from build123d import *

# Parameters (mm, degrees)
SKETCH1_R               = 25
BOSS_EXTRUDE1_DEPTH     = 249.6
SKETCH2_R               = 24.61
BOSS_EXTRUDE2_DEPTH     = 200
CUT_EXTRUDE1_DEPTH      = 451.987982102
CUT_EXTRUDE1_DEPTH_BACK = 451.987982102
SKETCH3_R               = 11


with BuildPart() as part:
    # Sketch1 → Boss-Extrude1 (new body)
    with BuildSketch(Plane(origin=(0, 0, 0), x_dir=(1, 0, 0), z_dir=(0, 1, 0))):
        with Locations(Location((0, 0, 0), (0, 0, 270))):
            Circle(SKETCH1_R)
    extrude(amount=BOSS_EXTRUDE1_DEPTH)

    # Sketch2 → Boss-Extrude2 (add)
    with BuildSketch(Plane(origin=(0, 249.6, 0), x_dir=(1, 0, 0), z_dir=(0, 1, 0))):
        with Locations(Location((0, 0, 0), (0, 0, 270))):
            Circle(SKETCH2_R)
    extrude(amount=BOSS_EXTRUDE2_DEPTH)

    # Sketch3 → Cut-Extrude1 (cut, two sides: drawn at the far end of the back side and taken through both)
    with BuildSketch(Plane(origin=(0, 0, 0), x_dir=(0, 0, -1), z_dir=(1, 0, 0)).offset(-CUT_EXTRUDE1_DEPTH_BACK)):
        with Locations((0, 299.6)):
            Circle(SKETCH3_R)
        with Locations((0, 399.6)):
            Circle(SKETCH3_R)
    extrude(amount=CUT_EXTRUDE1_DEPTH + CUT_EXTRUDE1_DEPTH_BACK, mode=Mode.SUBTRACT)


solid = part.part
Work out the finished part from the listing and answer in its coordinate system (mm). Round coordinates to 2 decimals unless told otherwise and drop trailing zeros. Loops run counter-clockwise (first coordinate to the right, second up) from the corner with the lowest first, then second, coordinate; pieces in that order, holes last. Notation, with made-up numbers: (75, 13.5) - (98, 13.5) arc R15 cw to (98, 23.5) - close; hole circle Ø3 at (23.25, 29.25). An arc over 180 degrees is marked (long way). Use one line per item in the form item = value. Start each with the question number.
(1) Find section D-D on y = 299.6. Determine the outline of the cut face in (x, z), and give its area (3 significant figures).
(2) Find section C-C on z = -19. Determine the outline of the cut face in (x, y), and give its area (3 significant figures).
(3) Find section B-B on x = 0. Determine the outline of the cut face in (y, z).
(4) Find section A-A on z = 0. Determine the outline of the cut face in (x, y), and give its area (3 significant figures).
(5) Determine the mould class of faces 1 (the face through (-0.345, 295.387, -10.161)), 2 (the face through (-9.43, 348.2, 22.73)), 3 (the face through (-16.6, 249.6, 18.4)) for opening direction Z: +Z half, -Z half, draft (parallel to the pull), parting line (faces both ways), or undercut.
(6) Flat-ended cylindrical pins translate along their axes: P1, Ø1, axis at y = 164.5, z = -17, coming from the +X side; P2, Ø6, axis at y = 148.5, z = -12.5, coming from the -X side; P3, Ø2, axis at y = 186, z = -3, coming from the -X side. Find the tip coordinate at first contact, or state that the pin passes through.
(7) Consider line 1 (Y direction, x = -2.5, z = 0); line 2 (Z direction, x = -1, y = 299.6); line 3 (Y direction, x = 5.5, z = -2.5). Determine where each line is inside the solid, lowest interval first.
Answer list:
q1.outline = (-22.01, -11) arc R24.61 ccw to (22.01, -11) - close; (-22.01, 11) - (22.01, 11) arc R24.61 ccw to start
q1.area = 857 mm^2
q2.outline = (-16.25, 0) - (16.25, 0) - (16.25, 249.6) - (15.64, 249.6) - (15.64, 449.6) - (-15.64, 449.6) - (-15.64, 249.6) - (-16.25, 249.6) - close
q2.area = 14,400 mm^2
q3.outline = (0, -25) - (249.6, -25) - (249.6, -24.61) - (449.6, -24.61) - (449.6, 24.61) - (249.6, 24.61) - (249.6, 25) - (0, 25) - close; hole circle Ø22 at (299.6, 0); hole circle Ø22 at (399.6, 0)
q4.outline = (-25, 0) - (25, 0) - (25, 249.6) - (24.61, 249.6) - (24.61, 288.6) - (-24.61, 288.6) - (-24.61, 249.6) - (-25, 249.6) - close; (-24.61, 310.6) - (24.61, 310.6) - (24.61, 388.6) - (-24.61, 388.6) - close; (-24.61, 410.6) - (24.61, 410.6) - (24.61, 449.6) - (-24.61, 449.6) - close
q4.area = 20,200 mm^2
q5.face_1 = undercut
q5.face_2 = parting line
q5.face_3 = draft
q6.P1 = 18.78
q6.P2 = -23.12
q6.P3 = -24.92
q7.line_1 = 0 to 288.6, 310.6 to 388.6, 410.6 to 449.6
q7.line_2 = -24.59 to -11, 11 to 24.59
q7.line_3 = 0 to 288.89, 310.31 to 388.89, 410.31 to 449.6
